Autodesk Inventor part; units mm, degrees
ref_plane "YZ Plane" through (0, 0, 0) normal (1, 0, 0) x (0, 1, 0)
ref_plane "XZ Plane" through (0, 0, 0) normal (0, 1, 0) x (-1, 0, 0)
ref_plane "XY Plane" through (0, 0, 0) normal (0, 0, 1) x (1, 0, 0)
sketch "Sketch1" plane through (0, 0, 0) normal (0, 0, 1) x (1, 0, 0)
  line L0 (0, 0) -> (20, 0) construction
  line L1 (20, 0) -> (20, 20) construction
  line L2 (20, 20) -> (0, 20) construction
  line L3 (0, 20) -> (0, 0) construction
  circle A0 centre (7.9375, 4.7625) radius 2
  circle A1 centre (7.9375, 4.7625) radius 0.75
  arc A2 (10.691, 11.6731) -> (5.9394, 4.676) centre (13.3396, 4.7625) ccw
  arc A3 (10.691, 11.6731) -> (9.9375, 4.7625) centre (38.5656, 5.1375) ccw
  dimension "d0" = 20
  dimension "d1" = 20
  dimension "d2" = 4
  dimension "d3" = 1.5
extrude "Extrusion1" add sketch "Sketch1" along normal blind 2 contours A0 A2 A3
fillet "Fillet2" radius 0.7 1 edges at (10.691, 11.6731, 1)
sketch "Sketch2" plane through (0, 0, 2) normal (0, 0, 1) x (1, 0, 0)
  arc A0 (5.9394, 4.676) -> (9.9375, 4.7625) centre (7.9375, 4.7625) ccw
  circle A1 centre (7.9375, 4.7625) radius 0.75
  arc A2 (10.3988, 10.2697) -> (9.9375, 4.7625) centre (38.5656, 5.1375) ccw
  arc A3 (9.331, 10.9836) -> (5.9394, 4.676) centre (13.3396, 4.7625) ccw
  arc A4 (10.3988, 10.2697) -> (9.331, 10.9836) centre (9.7101, 10.3952) ccw
  circle A5 centre (9.7101, 10.3952) radius 0.35
  point P0 (0, 0)
  dimension "d16" = 0.7
extrude "Extrusion2" add sketch "Sketch2" along normal blind 1.5 contours A5
sketch "Sketch3" plane through (0, 0, 0) normal (0, 0, -1) x (-1, 0, 0)
  arc A0 (-9.9375, 4.7625) -> (-5.9394, 4.676) centre (-7.9375, 4.7625) ccw
  circle A1 centre (-7.9375, 4.7625) radius 0.75
  arc A2 (-5.9394, 4.676) -> (-9.331, 10.9836) centre (-13.3396, 4.7625) ccw
  arc A3 (-9.9375, 4.7625) -> (-10.3988, 10.2697) centre (-38.5656, 5.1375) ccw
  arc A4 (-9.331, 10.9836) -> (-10.3988, 10.2697) centre (-9.7101, 10.3952) ccw
  circle A5 centre (-9.7101, 10.3952) radius 0.35
  point P0 (0, 0)
  dimension "d17" = 0.7
extrude "Extrusion3" add sketch "Sketch3" along normal blind 1.5 contours A5
properties material "Liga de Nickel-Copper 400"
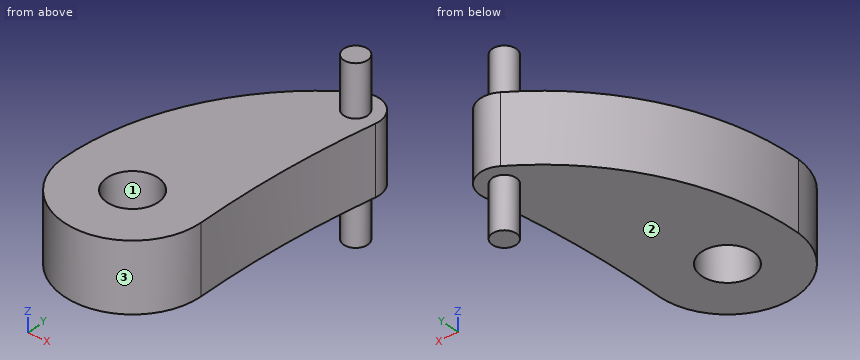
CAD build for the part. Positions are in the model's coordinates, mm. Face numbers are marked on the shaded views. Round coordinates to 2 decimals unless told otherwise and drop trailing zeros. Write each loop counter-clockwise with the first axis right and the second up, starting at its lowest first coordinate (ties: lowest second). Pieces come first, ordered by that corner, then holes. Notation, with made-up numbers: M 76,61 L 123,61 A24 cw 123,76 Z; hole C -27,71.5 d7. An arc over 180 degrees is marked long. Use a Markdown table: item, result. Add a question column.
1. Flat gauge pins, fed straight in: P1, Ø1, axis at x = 7.5, y = 7.5, coming from the -Z side; P2, Ø1.3, axis at x = 7.5, y = 8, coming from the +Z side; P3, Ø2, axis at y = 5, z = 1, coming from the +X side. Where does each tip first touch, or does it go through?
2. Slice it at B-B on y = 4.5. Give the cut face in (x, z).
3. Drill centre lines: probe 1 along Z at (x, y) = (7.7, 9.5); probe 2 along X at (y, z) = (5, 1.8); probe 3 along X at (y, z) = (4.25, 1.05). Where is each one in solid material? Low to high.
4. Slice it at C-C on z = 2.2. Give the cut face in (x, y).
5. Slice it at A-A on x = 7.85. Give the cut face in (y, z).
6. Pull direction X, two halves, no side cores. Call the marked faces 1, 2 and 3: released by +X, released by -X, zero draft, split by the parting line, or undercut.
7. Slice it at D-D on y = 8. Give the cut face in (x, z), then the cut area to 3 significant figures.
Reply:
| question | item | result |
|---|---|---|
| 1 | P1 | stops at z = 0 |
| 1 | P2 | stops at z = 2 |
| 1 | P3 | stops at x = 9.95 |
| 2 | outline | M 5.95,0 L 7.23,0 L 7.23,2 L 5.95,2 Z; M 8.64,0 L 9.92,0 L 9.92,2 L 8.64,2 Z |
| 3 | probe 1 | z = 0 to 2 |
| 3 | probe 2 | x = 5.94 to 7.23, 8.65 to 9.94 |
| 3 | probe 3 | x = 6 to 7.39, 8.49 to 9.87 |
| 4 | outline | C 9.71,10.4 d0.7 |
| 5 | outline | M 2.76,0 L 4.02,0 L 4.02,2 L 2.76,2 Z; M 5.51,0 L 9.73,0 L 9.73,2 L 5.51,2 Z |
| 6 | face 1 | undercut |
| 6 | face 2 | zero draft |
| 6 | face 3 | split by the parting line |
| 7 | outline | M 6.68,0 L 10.08,0 L 10.08,2 L 6.68,2 Z |
| 7 | area | 6.79 mm^2 |
